Could you check a few things on this model? Use its own coordinates, in mm. Give positions to 0.01 mm unless a question says otherwise; leave off trailing zeros. Loops run counter-clockwise (first coordinate to the right, second up) from the corner with the lowest first, then second, coordinate; pieces in that order, holes last. Notation, with made-up numbers: (74, 15.5) - (125, 15.5) arc R19 cw to (125, 50.5) - close; hole circle Ø1 at (-34.75, 44.5). An arc over 180 degrees is marked (long way). Write each question's results on one line, items separated by ' | '. Start each with the question number.
1) I want a section at B-B, the plane z = 38. Write out the boundary of the cut face in (x, y).
2) I want a section at A-A, the plane x = 0. Write out the boundary of the cut face in (y, z), and give its area (3 significant figures).
3) I'm going to push flat-ended pins straight in: pin 1 (2 mm diameter, centred on x = -2.5, z = 53.5, fed in from -Y); pin 2 (2 mm diameter, centred on x = -2.5, y = -0.5, fed in from +Z); pin 3 (1.5 mm diameter, centred on y = -2.5, z = -1.5, fed in from +X). Where does each tip first touch, or does it pass through?
4) If I drill on probe 1 along Z at (x, y) = (0, -2.5); probe 2 along Y at (x, z) = (3, 15.5); probe 3 along Y at (x, z) = (3.25, 6.5), over which ranges is the centre line in solid material (lowest first)? Write a range as [from, to].
from build123d import *

# Parameters (mm, degrees)
EXTRUDE_56_5_DEPTH  = 56.5
EXTRUDE_START       = -13
SKETCH_2_R          = 1.5
EXTRUDE_M3_13_DEPTH = 13
EXTRUDE_START_2     = 56.5
SKETCH_3_R          = 1.5
EXTRUDE_M3_9_DEPTH  = 9


with BuildPart() as part:
    # 草图1 → 六角柱_有效长56.5 (new body)
    with BuildSketch(Plane.XY):
        Polygon((3.464101615, 0), (1.732050808, 3), (-1.732050808, 3), (-3.464101615, 0), (-1.732050808, -3), (1.732050808, -3), align=None)
    extrude(amount=EXTRUDE_56_5_DEPTH)

    # 草图2 → 下端M3公头_长13 (add)
    with BuildSketch(Plane.XY.offset(EXTRUDE_START)):
        with Locations(Location((0, 0, 0), (0, 0, 180))):
            Circle(SKETCH_2_R)
    extrude(amount=EXTRUDE_M3_13_DEPTH)

    # 草图3 → 上端M3公头_长9 (add)
    with BuildSketch(Plane.XY.offset(EXTRUDE_START_2)):
        with Locations(Location((0, 0, 0), (0, 0, 180))):
            Circle(SKETCH_3_R)
    extrude(amount=EXTRUDE_M3_9_DEPTH)


solid = part.part
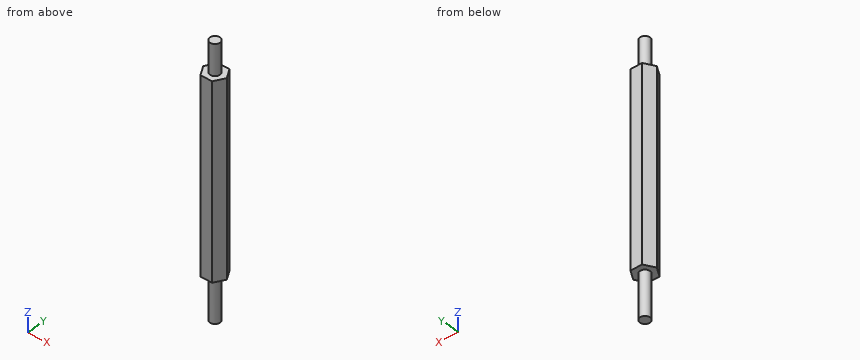
Answers:
1) outline: (-3.46, 0) - (-1.73, -3) - (1.73, -3) - (3.46, 0) - (1.73, 3) - (-1.73, 3) - close
2) outline: (-3, 0) - (-1.5, 0) - (-1.5, -13) - (1.5, -13) - (1.5, 0) - (3, 0) - (3, 56.5) - (1.5, 56.5) - (1.5, 65.5) - (-1.5, 65.5) - (-1.5, 56.5) - (-3, 56.5) - close | area: 405 mm2
3) pin 1: stops at y = -3 | pin 2: stops at z = 56.5 | pin 3: passes through
4) probe 1: z = [0, 56.5] | probe 2: y = [-0.8, 0.8] | probe 3: y = [-0.37, 0.37]
